```python
from build123d import *

# Parameters (mm, degrees)
F0_R     = 19.05
F2_DEPTH = 76.2
F1_W     = 25.4
F1_H     = 25.4
F3_DEPTH = 25.4


with BuildPart() as f2:
    # F0 (on Top) → F2 (new body, symmetric)
    with BuildSketch(Plane.XY):
        Circle(F0_R)
    extrude(amount=F2_DEPTH, both=True)

    # F1 (on Front) → F3 (cut, symmetric)
    with BuildSketch(Plane.XZ):
        with Locations((0, 52.537386)):
            Rectangle(F1_W, F1_H)
    extrude(amount=F3_DEPTH, both=True, mode=Mode.SUBTRACT)


solid = f2.part
```
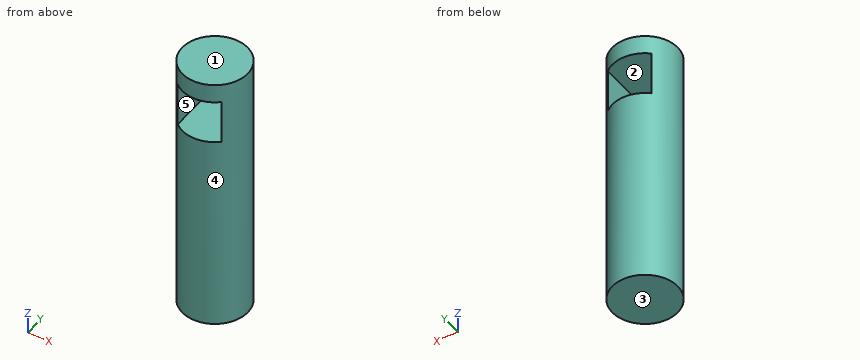
The model under review builds one solid part; all positions refer to its coordinate system, in mm. Face numbers are marked on the shaded views. A direction names the side the tool comes from. Coordinates: 2 decimals unless noted, no trailing zeros. Write each loop counter-clockwise with the first axis right and the second up, starting at its lowest first coordinate (ties: lowest second). Pieces come first, ordered by that corner, then holes. Notation, with made-up numbers: (1.5, 42) - (38.5, 42) arc R22 ccw to (38.5, 70) - close; hole circle Ø7 at (43.5, 71.25). An arc over 180 degrees is marked (long way). Answer in a Markdown table with one row per item. Add a question column.
Q1. Consider section B-B on y = 0. Give the boundary of the cut face in (x, z), then the cut area to 3 significant figures.
Q2. Consider section D-D on y = 16.5. Give the boundary of the cut face in (x, z), then the cut area to 3 significant figures.
Q3. For the marked faces 1 and 2, list the 3-axis set-ups (+Z, -Z, +X, -X, +Y, -Y) from which the entire face can be reached by the end or side of a thin tool; tool diameter is ignored.
Q4. To check wall thickness, follow line 1 along Z through (x, y) = (-8, 12); line 2 along X through (y, z) = (-11.5, 62.5); line 3 along Y through (x, z) = (-17, -30). State the ranges of each line that lie inside material, in increasing order. Write a range as from..to.
Q5. Draft analysis for pull direction X (two halves, no side actions). For the marked faces 3, 4 and 5, state which applies: +X half, -X half, draft (parallel to the pull), parting line (faces both ways), or undercut.
Q6. Consider section C-C on z = 47. Give the boundary of the cut face in (x, y), then the cut area to 3 significant figures.
Q7. Clearance check with flat-ended pins moving along their axes: pin 1 (12.5 mm diameter, centred on y = 4.5, z = 58, fed in from +X); pin 2 (12 mm diameter, centred on y = -11, z = -52.5, fed in from +X); pin 3 (3 mm diameter, centred on x = -4.5, z = -35, fed in from +Y); pin 4 (6 mm diameter, centred on x = -5.5, z = -17, fed in from +Y). State where each tip first meets the part, or that it passes through.
Q8. Consider section A-A on x = 0. Give the boundary of the cut face in (y, z), then the cut area to 3 significant figures.
Answers below:
| question | item | result |
|---|---|---|
| 1 | outline | (-19.05, -76.2) - (19.05, -76.2) - (19.05, 76.2) - (-19.05, 76.2) - close; hole (-12.7, 39.84) - (12.7, 39.84) - (12.7, 65.24) - (-12.7, 65.24) - close |
| 1 | area | 5,160 mm² |
| 2 | outline | (-9.52, -76.2) - (9.52, -76.2) - (9.52, 39.84) - (-9.52, 39.84) - close; (-9.52, 65.24) - (9.52, 65.24) - (9.52, 76.2) - (-9.52, 76.2) - close |
| 2 | area | 2,420 mm² |
| 3 | face 1 | +Z, +X, -X, +Y, -Y |
| 3 | face 2 | +Y, -Y |
| 4 | line 1 | -76.2..39.84, 65.24..76.2 |
| 4 | line 2 | -15.19..-12.7, 12.7..15.19 |
| 4 | line 3 | -8.6..8.6 |
| 5 | face 3 | draft |
| 5 | face 4 | parting line |
| 5 | face 5 | undercut |
| 6 | outline | (-12.7, -14.2) - (-12.7, 14.2) arc R19.05 ccw to start; (12.7, -14.2) arc R19.05 ccw to (12.7, 14.2) - close |
| 6 | area | 250 mm² |
| 7 | pin 1 | x = 19.05 |
| 7 | pin 2 | x = 18.38 |
| 7 | pin 3 | y = 18.81 |
| 7 | pin 4 | y = 18.89 |
| 8 | outline | (-19.05, -76.2) - (19.05, -76.2) - (19.05, 39.84) - (-19.05, 39.84) - close; (-19.05, 65.24) - (19.05, 65.24) - (19.05, 76.2) - (-19.05, 76.2) - close |
| 8 | area | 4,840 mm² |
